Geometry: final body of the model. Coordinates: model frame, mm. A direction names the side the tool comes from. Give positions to 0.01 mm unless a question says otherwise; leave off trailing zeros. Order: outer loops, then holes, each group sorted by start corner. A loop starts at its lowest first (then second) coordinate and runs counter-clockwise, first axis right, second up. Notation, with made-up numbers: (67.5, -15.75) -> (83.5, -15.75) arc R20 cw to (83.5, 2.25) -> close; hole circle Ø8 at (3.25, 12). An arc over 180 degrees is marked (long way). One line per item, written item: value. Start each with the question number.
```python
from build123d import *

# Parameters (mm, degrees)
SKETCH_1_R                 = 54
SKETCH_1_R_2               = 15
EXTRUDE_1_DEPTH            = 20
FILLET_1_R                 = 10
SKETCH_2_R                 = 37.711489045
SKETCH_2_R_2               = 25.889208159
CUT_EXTRUDE_1_DEPTH        = 8
CHAMFER_1_SIZE             = 5
CHAMFER_1_OF_MIRROR_4_SIZE = 5


with BuildPart() as part:
    # 草图1 → 凸台-拉伸1 (new, symmetric)
    with BuildSketch(Plane(origin=(0, 0, 0), x_dir=(0, 0, -1), z_dir=(1, 0, 0))):
        Circle(SKETCH_1_R)
        Circle(SKETCH_1_R_2, mode=Mode.SUBTRACT)
    extrude(amount=EXTRUDE_1_DEPTH, both=True)

    # 圆角1
    fillet_1_edges = [part.edges().sort_by_distance(p)[0] for p in [
        (-20, 0, 54),
        (20, 0, 54),
    ]]
    fillet(fillet_1_edges, radius=FILLET_1_R)

    # 草图2 → 切除-拉伸1 (cut)
    with BuildSketch(Plane(origin=(20, 0, 0), x_dir=(0, 0, -1), z_dir=(1, 0, 0))):
        Circle(SKETCH_2_R)
        Circle(SKETCH_2_R_2, mode=Mode.SUBTRACT)
    cut_extrude_1 = extrude(amount=-CUT_EXTRUDE_1_DEPTH, mode=Mode.SUBTRACT)

    # 倒角1
    chamfer_1_edges = [part.edges().sort_by_distance(p)[0] for p in [
        (20, 0, 37.711489045),
        (20, 0, 25.889208159),
    ]]
    chamfer(chamfer_1_edges, length=CHAMFER_1_SIZE)

    # 镜向4: 切除-拉伸1 across plane
    add(cut_extrude_1.mirror(Plane(origin=(0, 0, 0), x_dir=(0, 0, 1), z_dir=(1, 0, 0))), mode=Mode.SUBTRACT)

    # 倒角1 of 镜向4
    chamfer_1_of_mirror_4_edges = [part.edges().sort_by_distance(p)[0] for p in [
        (-20, 0, 37.711489045),
        (-20, 0, 25.889208159),
    ]]
    chamfer(chamfer_1_of_mirror_4_edges, length=CHAMFER_1_OF_MIRROR_4_SIZE)


solid = part.part
```
1. Pin query (flat end, axial travel): P1, Ø2, axis at x = 2.5, z = -38.5, coming from the +Y side; P2, Ø10, axis at x = 5.5, z = -41.5, coming from the +Y side; P3, Ø1.5, axis at y = 34.5, z = -35, coming from the -X side. Return the tip coordinate at first contact, or that it passes through.
2. Material intervals for L1, parallel to Y at x = 12.75, z = 0; L2, parallel to Z at x = -16, y = -17; L3, parallel to Y at x = -13.2, z = 0, sorted ascending. Write a range as [from, to].
3. Access query for faces 4 (the cylindrical face through (-13.52, 11.33, -35.97)), 5 (the cylindrical face through (13.52, 11.33, -35.97)), 6 (the flat face through (20, 43, 3)). Directions: +Z, -Z, +X, -X, +Y, -Y. A direction counts if a zero-diameter tool reaches every point of the face in a straight line with its end or side. Return the directions, or none.
4. Cut plane A-A, the plane x = 0. Return loops of the section in (y, z).
5. Draft query along Y for faces 1 (the flat face through (20, -14, -9)), 2 (the cylindrical face through (0.14, -52.716, 11.706)), 3 (the cylindrical face through (-13.521, -25.274, 5.612)). Return one class per face: pulls with the +Y half, pulls with the -Y half, needs draft (parallel to the pull), parting line crosses it, or undercut.
Answers follow:
1. P1: stops at y = 38.86
1. P2: stops at y = 39.8
1. P3: stops at x = -18.98
2. L1: y = [-53.61, -37.71], [-25.89, -15], [15, 25.89], [37.71, 53.61]
2. L2: z = [-49.14, -34.78], [-18.18, 18.18], [34.78, 49.14]
2. L3: y = [-53.47, -37.71], [-25.89, -15], [15, 25.89], [37.71, 53.47]
3. face 4: -X
3. face 5: +X
3. face 6: +Z, -Z, +X, +Y, -Y
4. outline: circle Ø108 at (0, 0); hole circle Ø30 at (0, 0)
5. face 1: needs draft
5. face 2: parting line crosses it
5. face 3: undercut
